Here's the drawing with two shaded views (mm, measured from the low corner). I have some questions. A direction names the side the tool comes from. Round coordinates to 2 decimals unless told otherwise and drop trailing zeros. Loops run counter-clockwise (first coordinate to the right, second up) from the corner with the lowest first, then second, coordinate; pieces in that order, holes last. Notation, with made-up numbers: M 18,-8 L 31,-8 A30 ccw 31,21 Z; hole C 86.25,65 d11. An arc over 180 degrees is marked long. One line per item, written item: value. Start each with the question number.
Q1. I'm going to push flat-ended pins straight in: pin 1 Ø3.5 at (x, z) = (19, 2.5) entering from -Y; pin 2 Ø19.5 at (x, y) = (25.5, 9.5) entering from +Z. Where does each tip first touch, or does it pass through?
Q2. Imagine slicing it at D-D (x = 56.2). Please give me the cut outline in (y, z).
Q3. Imagine slicing it at B-B (z = 6.5). Please give me the cut outline in (x, y), then the cut area to 3 significant figures.
Q4. Please list where these lines run through material, in increasing order: line 1 along X through (y, z) = (47, 1.25); line 2 along X through (y, z) = (31, 3.75); line 3 along X through (y, z) = (25, 8.5).
Q5. Imagine slicing it at A-A (y = 37). Please give me the cut outline in (x, z).
Q6. Thinking about a two-plate mould opening in X: for the marked faces 3, 4, 5 and 6, which applies, released by +X, released by -X, zero draft, split by the parting line, or undercut?
Q7. Which directions (+Z, -Z, +X, -X, +Y, -Y) give clear straight access to the entire face, cutting with the end or side of a thin tool? Please do the marked faces 1 and 2.
Q8. Imagine slicing it at C-C (x = 25). Please give me the cut outline in (y, z), then the cut area to 3 significant figures.
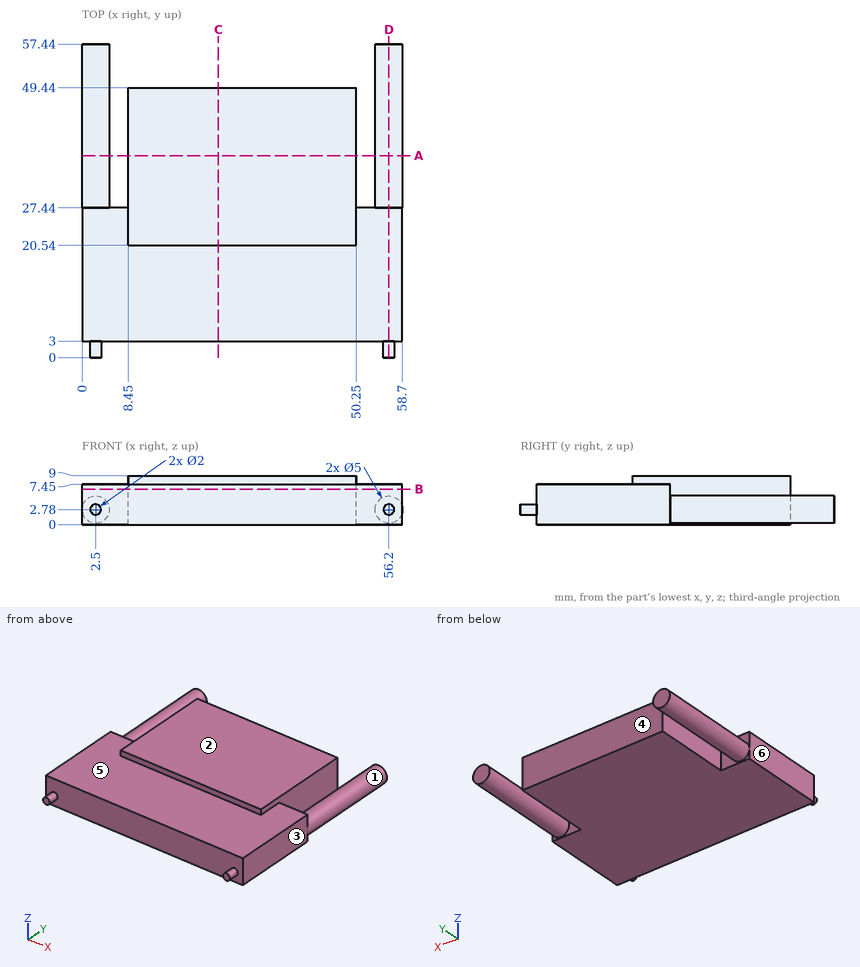
Report:
1. pin 1: stops at y = 3
1. pin 2: stops at z = 7.45
2. outline: M 0,1.78 L 3,1.78 L 3,0 L 27.44,0 L 27.44,0.28 L 57.44,0.28 L 57.44,5.28 L 27.44,5.28 L 27.44,7.45 L 3,7.45 L 3,3.78 L 0,3.78 Z
3. outline: M 0,3 L 58.7,3 L 58.7,27.44 L 50.25,27.44 L 50.25,49.44 L 8.45,49.44 L 8.45,27.44 L 0,27.44 Z
3. area: 2,350 mm²
4. line 1: x = 0.52 to 4.48, 8.45 to 50.25, 54.22 to 58.18
4. line 2: x = 0.2 to 4.8, 8.45 to 50.25, 53.9 to 58.5
4. line 3: x = 8.45 to 50.25
5. outline: C 2.5,2.78 d5; M 8.45,0 L 50.25,0 L 50.25,9 L 8.45,9 Z; C 56.2,2.78 d5
6. face 3: released by +X
6. face 4: undercut
6. face 5: zero draft
6. face 6: released by -X
7. face 1: +Y
7. face 2: +Z, +X, -X, +Y, -Y
8. outline: M 3,0 L 49.44,0 L 49.44,9 L 20.54,9 L 20.54,7.45 L 3,7.45 Z
8. area: 391 mm²
